```python
from build123d import *

# Parameters (mm, degrees)
SKETCH1_W            = 42
SKETCH1_H            = 42
BOSS_EXTRUDE1_DEPTH  = 3
M3_CLEARANCE_HOLE1_D = 3.6
SKETCH4_R            = 12
CUT_EXTRUDE1_DEPTH   = 30.849623113
BOSS_EXTRUDE2_START  = -34
SKETCH5_R            = 4
BOSS_EXTRUDE2_DEPTH  = 20
SKETCH6_W            = 42
SKETCH6_H            = 20
BOSS_EXTRUDE3_DEPTH  = 3
SKETCH7_W            = 4.75
SKETCH7_H            = 62
BOSS_EXTRUDE4_DEPTH  = 3
BOSS_EXTRUDE5_START  = -7
BOSS_EXTRUDE5_DEPTH  = 9
SKETCH13_W           = 13.25
SKETCH13_H           = 20
BOSS_EXTRUDE6_DEPTH  = 3
M5_CLEARANCE_HOLE1_D = 5.5
CHAMFER1_SIZE        = 4
MOVE_FACE1_BY        = 4


with BuildPart() as part:
    # Sketch1 → Boss-Extrude1 (new body)
    with BuildSketch(Plane(origin=(0, 0, 0), x_dir=(1, 0, 0), z_dir=(0, 1, 0))):
        Rectangle(SKETCH1_W, SKETCH1_H)
    extrude(amount=BOSS_EXTRUDE1_DEPTH)

    # M3 Clearance Hole1 (through all)
    with Locations(Plane(origin=(0, 3, 0), x_dir=(1, 0, 0), z_dir=(0, 1, 0))):
        with Locations((-15.5, 15.5), (-15.5, -15.5), (15.5, -15.5), (15.5, 15.5)):
            Hole(M3_CLEARANCE_HOLE1_D / 2)

    # Sketch4 → Cut-Extrude1 (cut, through all)
    with BuildSketch(Plane(origin=(0, 3, 0), x_dir=(1, 0, 0), z_dir=(0, 1, 0))):
        with Locations(Location((0, 0, 0), (0, 0, 270))):
            Circle(SKETCH4_R)
    extrude(amount=-CUT_EXTRUDE1_DEPTH, mode=Mode.SUBTRACT)

    # Sketch6 → Boss-Extrude3 (add)
    with BuildSketch(Plane(origin=(0, 0, 0), x_dir=(1, 0, 0), z_dir=(0, 1, 0))):
        with Locations((0, 31)):
            Rectangle(SKETCH6_W, SKETCH6_H)
    extrude(amount=BOSS_EXTRUDE3_DEPTH)

    # Sketch7 → Boss-Extrude4 (add)
    with BuildSketch(Plane(origin=(0, 0, 0), x_dir=(1, 0, 0), z_dir=(0, 1, 0))):
        with Locations((-23.375, 10)):
            Rectangle(SKETCH7_W, SKETCH7_H)
        with Locations((23.375, 10)):
            Rectangle(SKETCH7_W, SKETCH7_H)
    extrude(amount=BOSS_EXTRUDE4_DEPTH)

    # Sketch8 → Boss-Extrude5 (add)
    with BuildSketch(Plane.XY.offset(-34).offset(BOSS_EXTRUDE5_START)):
        with BuildLine():
            Line((-22.46, 17.075), (-22.46, 3))
            Line((-22.46, 3), (-15.738219121, 3))
            ThreePointArc((-15.738219121, 3), (-19.033415417, 6.886369723), (-15.96, 10.95039555))
            Line((-15.96, 10.95039555), (-15.96, 17.075))
            Line((-15.96, 17.075), (-22.46, 17.075))
        make_face()
        with BuildLine():
            ThreePointArc((-13.96, 10.95039555), (-10.886584583, 6.886369723), (-14.181780879, 3))
            Line((-14.181780879, 3), (-7.46, 3))
            Line((-7.46, 3), (-7.46, 17.075))
            Line((-7.46, 17.075), (-13.96, 17.075))
            Line((-13.96, 17.075), (-13.96, 10.95039555))
        make_face()
    boss_extrude5 = extrude(amount=BOSS_EXTRUDE5_DEPTH)

    # Sketch10 → M3 Clearance Hole2 (revolve, cut)
    with BuildSketch(Plane(origin=(-7.46, 14.012697775, -36.5), x_dir=(0, 0, -1), z_dir=(0, 1, 0))):
        Polygon((0, 0), (0, 7.371463052), (1.7, 6.35), (1.7, 0), align=None)
    m3_clearance_hole2 = revolve(axis=Axis((-1.11, 14.012697775, -36.5), (-1, 0, 0)), mode=Mode.SUBTRACT)

    # Mirror2: Boss-Extrude5, M3 Clearance Hole2 across plane
    add(boss_extrude5.mirror(Plane(origin=(0, 0, 0), x_dir=(0, 0, 1), z_dir=(1, 0, 0))))
    add(m3_clearance_hole2.mirror(Plane(origin=(0, 0, 0), x_dir=(0, 0, 1), z_dir=(1, 0, 0))), mode=Mode.SUBTRACT)

    # Sketch13 → Boss-Extrude6 (add)
    with BuildSketch(Plane(origin=(0, 3, 0), x_dir=(1, 0, 0), z_dir=(0, 1, 0))):
        with Locations((-32.375, 31)):
            Rectangle(SKETCH13_W, SKETCH13_H)
        with Locations((32.375, 31)):
            Rectangle(SKETCH13_W, SKETCH13_H)
    extrude(amount=-BOSS_EXTRUDE6_DEPTH)

    # M5 Clearance Hole1 (through all)
    with Locations(Plane(origin=(0, 3, 0), x_dir=(1, 0, 0), z_dir=(0, 1, 0))):
        with Locations((0, 31), (-31.5, 31), (31.5, 31)):
            Hole(M5_CLEARANCE_HOLE1_D / 2)

    # Chamfer1
    chamfer1_edges = [part.edges().sort_by_distance(p)[0] for p in [
        (22.46, 3, -36.5),
        (-22.46, 3, -36.5),
    ]]
    chamfer(chamfer1_edges, length=CHAMFER1_SIZE)

    # Move Face1: a face moved outward by 4.0
    extrude(part.faces().sort_by_distance((0, 0, -14.610959183))[0], amount=MOVE_FACE1_BY, dir=(0, -1, 0))


with BuildPart() as body_2:
    # Sketch5 → Boss-Extrude2 (new body)
    with BuildSketch(Plane.XY.offset(BOSS_EXTRUDE2_START)):
        with Locations((-14.96, 7)):
            Circle(SKETCH5_R)
    extrude(amount=-BOSS_EXTRUDE2_DEPTH)


solid = part.part
```
Source: CAD feature listing. Evaluate the final solid. Frame: model axes, mm. A direction names the side the tool comes from. Coordinates: 2 decimals unless noted, no trailing zeros. Write each loop counter-clockwise with the first axis right and the second up, starting at its lowest first coordinate (ties: lowest second). Pieces come first, ordered by that corner, then holes. Notation, with made-up numbers: (79, 27) - (137, 27) arc R22 cw to (137, 55) - close; hole circle Ø3 at (2.5, 76.25). An arc over 180 degrees is marked (long way). Answer as a JSON object with one key per item and string values.
Q1. Section query B-B, the plane z = -15.5. Output: boundary loops of the cut face in (x, y).
Ans:
{"outline": "(-25.75, -4) - (-17.3, -4) - (-17.3, 3) - (-25.75, 3) - close; (-13.7, -4) - (13.7, -4) - (13.7, 3) - (-13.7, 3) - close; (17.3, -4) - (25.75, -4) - (25.75, 3) - (17.3, 3) - close"}
Q2. Section query D-D, the plane y = 5. Output: boundary loops of the cut face in (x, z), plus the area to 3 significant figures.
Ans:
{"outline": "(-24.46, -41) - (-18.51, -41) - (-18.51, -32) - (-24.46, -32) - close; (-11.41, -41) - (-7.46, -41) - (-7.46, -32) - (-11.41, -32) - close; (7.46, -41) - (11.41, -41) - (11.41, -32) - (7.46, -32) - close; (18.51, -41) - (24.46, -41) - (24.46, -32) - (18.51, -32) - close", "area": "178 mm2"}
Q3. Set-up query: faces 1 (the flat face through (-25.75, 0, 0)), 2 (the cylindrical face through (-19.03, 6.81, -36.56)), 3 (the flat face through (-22.46, 12, -37)). Return all of +Z, -Z, +X, -X, +Y, -Y with unobstructed straight access to the full face (end or side cutting, diameter ignored); none if empty.
Ans:
{"face 1": "+Z, -X, +Y, -Y", "face 2": "+Z, -Z", "face 3": "+Z, -Z, -X, +Y"}
Q4. First-contact query: pin 1 Ø1.5 at (y, z) = (3.5, -7) entering from -X; pin 2 Ø4 at (y, z) = (2.5, -1.5) entering from +X; pin 3 Ø5 at (y, z) = (13.5, -37.5) entering from -X. Flat tips, straight axial feed; report the tip coordinate or a pass-through.
Ans:
{"pin 1": "stops at x = -25.75", "pin 2": "stops at x = 25.75", "pin 3": "stops at x = -22.46"}
Q5. Section query C-C, the plane x = -31.5. Output: boundary loops of the cut face in (y, z), plus the area to 4 significant figures.
Ans:
{"outline": "(-4, -41) - (3, -41) - (3, -33.75) - (-4, -33.75) - close; (-4, -28.25) - (3, -28.25) - (3, -21) - (-4, -21) - close", "area": "101.5 mm2"}
Q6. Section query A-A, the plane x = 0. Output: boundary loops of the cut face in (y, z), plus the area to 4 significant figures.
Ans:
{"outline": "(-4, -41) - (3, -41) - (3, -33.75) - (-4, -33.75) - close; (-4, -28.25) - (3, -28.25) - (3, -12) - (-4, -12) - close; (-4, 12) - (3, 12) - (3, 21) - (-4, 21) - close", "area": "227.5 mm2"}
Q7. Material intervals for line 1 (X direction, y = -1.05, z = -31); line 2 (X direction, y = -2.75, z = 15.5); line 3 (Z direction, x = -15.5, y = 2.1), sorted ascending. Write a range as [from, to].
Ans:
{"line 1": "x = [-39, -34.25], [-28.75, -2.75], [2.75, 28.75], [34.25, 39]", "line 2": "x = [-25.75, -17.3], [-13.7, 13.7], [17.3, 25.75]", "line 3": "z = [-41, -17.3], [-13.7, 13.7], [17.3, 21]"}
